Check sheet for the drawn part. Datum: minimum x, y, z corner. Units: mm. A direction names the side the tool comes from. Round coordinates to 2 decimals unless told otherwise and drop trailing zeros. Write each loop counter-clockwise with the first axis right and the second up, starting at its lowest first coordinate (ties: lowest second). Pieces come first, ordered by that corner, then holes. Notation, with made-up numbers: (5.5, -9) -> (15.5, -9) arc R32 ccw to (15.5, 27) -> close; hole circle Ø5 at (39, 52.25). An arc over 180 degrees is marked (long way). One line per item, written item: value. Start each with the question number.
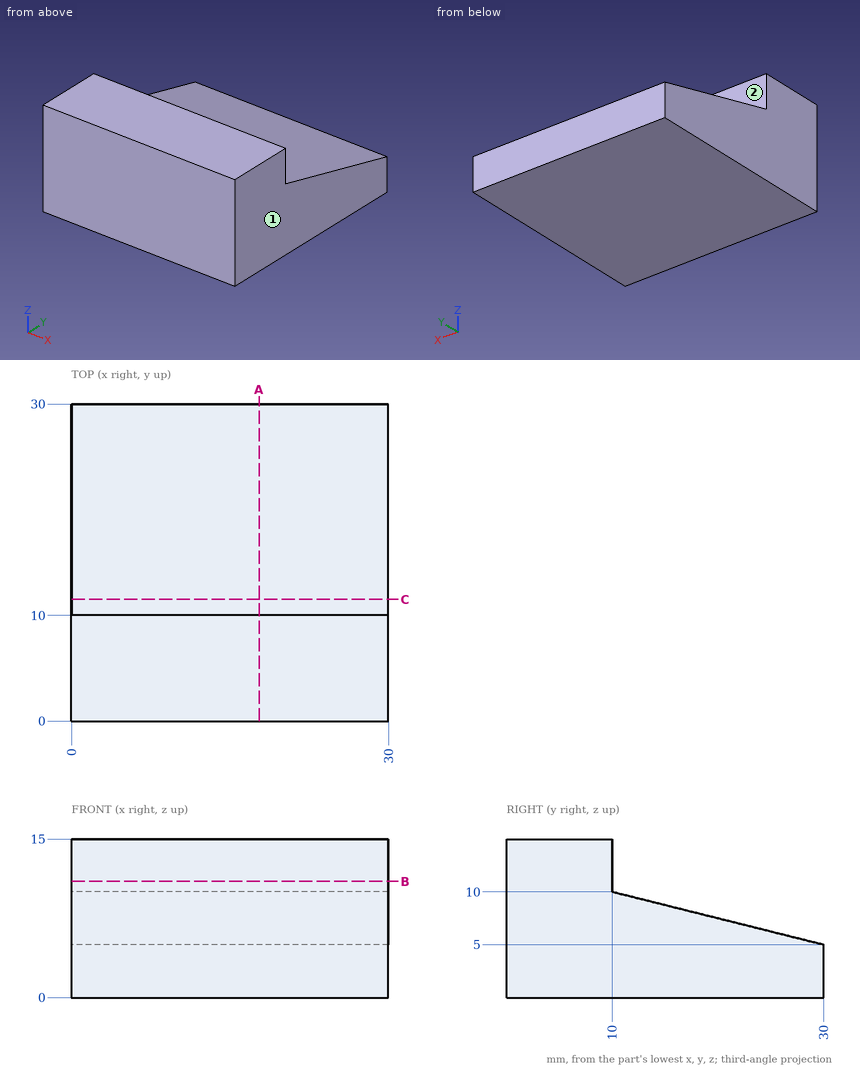
1. Cross-section at C-C (y = 11.5). Record the cut outline in (x, z) (3 decimals).
2. Cross-section at B-B (z = 11). Record the cut outline in (x, y).
3. Material ranges on probe 1 along Y at (x, z) = (22, 12.25); probe 2 along Z at (x, y) = (26.25, 13); probe 3 along Z at (x, y) = (14.75, 26), recorded low to high.
4. Cross-section at A-A (x = 17.75). Record the cut outline in (y, z), plus the area to 3 significant figures.
5. Access from +Z, -Z, +X, -X, +Y, -Y to the whole of each face (thin tool, end or side, straight path). Record for the marked faces 1 and 2.
6. Depth check by flat-ended pin: pin 1 Ø1.5 at (x, z) = (14.5, 13.5) entering from +Y; pin 2 Ø4 at (x, y) = (17.5, 25.5) entering from +Z (3 decimals); pin 3 Ø2 at (x, y) = (8.5, 18.5) entering from +Z (3 decimals). Enter the tip coordinate at first touch or a pass-through.
Working result:
1. outline: (0, 0) -> (30, 0) -> (30, 9.625) -> (0, 9.625) -> close
2. outline: (0, 0) -> (30, 0) -> (30, 10) -> (0, 10) -> close
3. probe 1: y = 0 to 10
3. probe 2: z = 0 to 9.25
3. probe 3: z = 0 to 6
4. outline: (0, 0) -> (30, 0) -> (30, 5) -> (10, 10) -> (10, 15) -> (0, 15) -> close
4. area: 300 mm^2
5. face 1: +Z, -Z, +X, +Y, -Y
5. face 2: +Z, +X, -X, +Y
6. pin 1: stops at y = 10
6. pin 2: stops at z = 6.625
6. pin 3: stops at z = 8.125
